The listing builds one solid part. Answer for the finished solid, in the listing's coordinates (mm). Face numbers are marked on the shaded views. A direction names the side the tool comes from. Coordinates: 2 decimals unless noted, no trailing zeros. Order: outer loops, then holes, each group sorted by start corner. A loop starts at its lowest first (then second) coordinate and runs counter-clockwise, first axis right, second up.
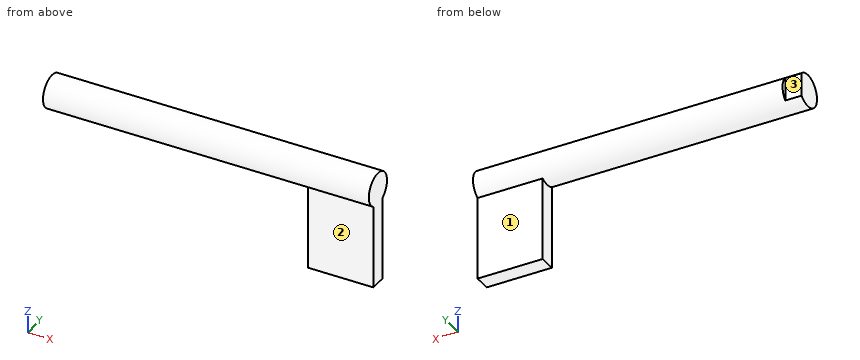
Autodesk Inventor part; units mm, degrees
ref_plane "YZ Plane" through (0, 0, 0) normal (1, 0, 0) x (0, 1, 0)
ref_plane "XZ Plane" through (0, 0, 0) normal (0, 1, 0) x (-1, 0, 0)
ref_plane "XY Plane" through (0, 0, 0) normal (0, 0, 1) x (1, 0, 0)
sketch "Sketch1" plane through (0, 0, 0) normal (1, 0, 0) x (0, 1, 0)
  circle A0 centre (0, 0) radius 6.35
  dimension "d0" = 12.7
extrude "Extrusion1" add sketch "Sketch1" along normal blind 127
sketch "Sketch2" plane through (127, 0, 0) normal (1, 0, 0) x (0, 0, -1)
  circle A0 centre (0, 0) radius 6.35
  line L0 (0, 3.175) -> (38.1, 3.175)
  line L1 (38.1, 3.175) -> (38.1, -3.175)
  line L2 (38.1, -3.175) -> (0, -3.175)
  line L3 (0, -3.175) -> (0, 3.175)
  dimension "d3" = 12.7
  dimension "d4" = 6.35
  dimension "d5" = 3.175
  dimension "d6" = 38.1
  dimension "d7" = 0
extrude "Extrusion2" add sketch "Sketch2" against normal blind 25.4 contours A0 L2 L3 L0 | A0 L0 L1 L2 picked at (2.1167, 0)
sketch "Sketch3" plane through (0, 0, 0) normal (-1, 0, 0) x (0, 0, 1)
  circle A0 centre (0, 0) radius 6.35
  circle A1 centre (0, 0) radius 6.35
  line L0 (-4.5348, 4.445) -> (4.5348, 4.445)
  line L1 (-5.4993, 3.175) -> (-38.1, 3.175)
  dimension "d10" = 4.445
extrude "Extrusion3" cut sketch "Sketch3" against normal blind 6.35 contours L0 A0 picked at (-0.24, 5.0664)
properties part number "StressTestPart"
(1) Find section A-A on y = 0. Determine the outline of the cut face in (x, z), then the cut area to 3 significant figures.
(2) Find section C-C on z = -30.5. Determine the outline of the cut face in (x, y) (3 decimals).
(3) Find section B-B on x = 56. Determine the outline of the cut face in (y, z), then the cut area to 3 significant figures.
(4) Find section D-D on x = 103. Determine the outline of the cut face in (y, z) (3 decimals), then the cut area to 3 significant figures.
(5) Given pin 1 Ø2 at (x, y) = (114, -2.5) entering from +Z; pin 2 Ø1 at (x, y) = (48, -2.5) entering from -Z; pin 3 Ø7.5 at (x, z) = (116.5, -17) entering from +Y (3 decimals), each flat-ended and moving along its own axis, determine where each tip first touches the part or whether it passes through.
(6) A tool of negligible diameter and unlimited length cuts with its end or side. For the marked faces 1, 2 and 3, from which of +Z, -Z, +X, -X, +Y, -Y can it reach the whole face along a straight path? Write none if from no direction.
(7) Find the intervals of material crossed by probe 1 along X at (y, z) = (-1.75, -12.5); probe 2 along Y at (x, z) = (96, -5.5); probe 3 along Z at (x, y) = (13, -0.5), in increasing order.
Resolved:
1. outline: (0, -6.35) - (101.6, -6.35) - (101.6, -38.1) - (127, -38.1) - (127, 6.35) - (0, 6.35) - close
1. area: 2,420 mm2
2. outline: (101.6, -3.175) - (127, -3.175) - (127, 3.175) - (101.6, 3.175) - close
3. outline: circle Ø12.7 at (0, 0)
3. area: 127 mm2
4. outline: (-3.175, -38.1) - (3.175, -38.1) - (3.175, -5.499) arc R6.35 ccw (long way) to (-3.175, -5.499) - close
4. area: 330 mm2
5. pin 1: stops at z = 6.17
5. pin 2: stops at z = -6.03
5. pin 3: stops at y = 3.175
6. face 1: -Z, +X, -X, +Y
6. face 2: -Z, +X, -X, -Y
6. face 3: +Z, -Z, -X, +Y
7. probe 1: x = 101.6 to 127
7. probe 2: y = -3.17 to 3.17
7. probe 3: z = -6.33 to 6.33
